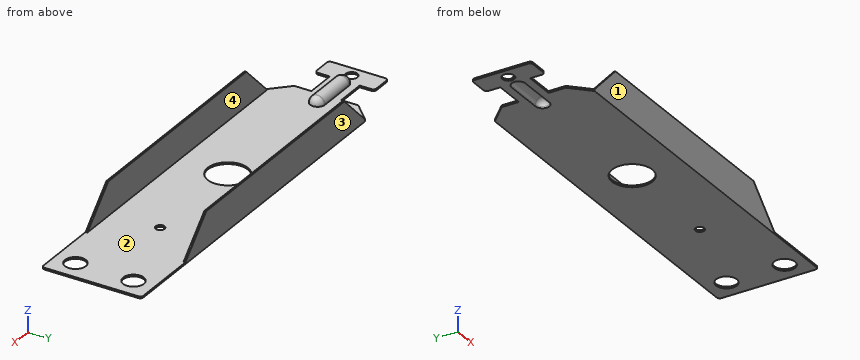
from build123d import *

# Parameters (mm, degrees)
F0_R     = 4.445
F0_R_2   = 8.5725
F0_R_3   = 1.905
F0_W     = 17.4625
F0_H     = 12.7
F0_W_2   = 12.7
F1_DEPTH = 0.762
F3_DEPTH = 0.762
F4_W     = 16.51
F4_H     = 2.921
F5_DEPTH = 25.4
F6_ANGLE = 180


# Not quite as in the source:
# - a pattern or mirror of a feature is missing from the dataset's text; its kind, count and spacing are read off the source's solid


with BuildPart() as f1:
    # F0 (on Top) → F1 (new body)
    with BuildSketch(Plane.XY):
        with BuildLine():
            Line((79.6925, 21.2725), (-73.3425, 21.2725))
            Line((-73.3425, 21.2725), (-80.9625, 13.6525))
            Line((-80.9625, 13.6525), (-80.9625, 6.35))
            Line((-80.9625, 6.35), (-63.5, 6.35))
            Line((-63.5, 6.35), (-63.5, -6.35))
            Line((-63.5, -6.35), (-80.9625, -6.35))
            Line((-80.9625, -6.35), (-80.9625, -13.6525))
            Line((-80.9625, -13.6525), (-73.3425, -21.2725))
            Line((-73.3425, -21.2725), (79.6925, -21.2725))
            ThreePointArc((79.6925, -21.2725), (80.5905256121, -20.9005256121), (80.9625, -20.0025))
            Line((80.9625, -20.0025), (80.9625, 20.0025))
            ThreePointArc((80.9625, 20.0025), (80.5905256121, 20.9005256121), (79.6925, 21.2725))
        make_face()
        with Locations((72.0725, -12.3825)):
            Circle(F0_R, mode=Mode.SUBTRACT)
        with Locations((-13.0175, 0)):
            Circle(F0_R_2, mode=Mode.SUBTRACT)
        with Locations((33.655, 0)):
            Circle(F0_R_3, mode=Mode.SUBTRACT)
        with Locations((72.0725, 12.3825)):
            Circle(F0_R, mode=Mode.SUBTRACT)
        with Locations((-72.23125, 0)):
            Rectangle(F0_W, F0_H)
        with Locations((-87.3125, 0)):
            Rectangle(F0_W_2, F0_H)
        with BuildLine():
            Line((-93.6625, -6.35), (-93.6625, 6.35))
            Line((-93.6625, 6.35), (-98.425, 6.35))
            Line((-98.425, 6.35), (-98.425, 2.54))
            ThreePointArc((-98.425, 2.54), (-96.6289487758, 1.7960512242), (-95.885, 0))
            ThreePointArc((-95.885, 0), (-96.6289487758, -1.7960512242), (-98.425, -2.54))
            Line((-98.425, -2.54), (-98.425, -6.35))
            Line((-98.425, -6.35), (-93.6625, -6.35))
        make_face()
        with BuildLine():
            Line((-98.425, 6.35), (-93.6625, 6.35))
            Line((-93.6625, 6.35), (-93.6625, 11.43))
            ThreePointArc((-93.6625, 11.43), (-94.0344743879, 12.3280256121), (-94.9325, 12.7))
            Line((-94.9325, 12.7), (-101.9175, 12.7))
            ThreePointArc((-101.9175, 12.7), (-102.8155256121, 12.3280256121), (-103.1875, 11.43))
            Line((-103.1875, 11.43), (-103.1875, -11.43))
            ThreePointArc((-103.1875, -11.43), (-102.8155256121, -12.3280256121), (-101.9175, -12.7))
            Line((-101.9175, -12.7), (-94.9325, -12.7))
            ThreePointArc((-94.9325, -12.7), (-94.0344743879, -12.3280256121), (-93.6625, -11.43))
            Line((-93.6625, -11.43), (-93.6625, -6.35))
            Line((-93.6625, -6.35), (-98.425, -6.35))
            Line((-98.425, -6.35), (-98.425, -2.54))
            ThreePointArc((-98.425, -2.54), (-100.965, 0), (-98.425, 2.54))
            Line((-98.425, 2.54), (-98.425, 6.35))
        make_face()
    extrude(amount=F1_DEPTH)

    # F2 (on face) → F3 (join)
    with BuildSketch(Plane.XZ.offset(21.2725)):
        Polygon((-58.9740902063, 15.1304097937), (-73.3425, 0.762), (50.6443195874, 0.762), (36.2759097937, 15.1304097937), align=None)
    f3 = extrude(amount=-F3_DEPTH)

    # F3_copies: F3 across plane
    add(f3.mirror(Plane.ZX))

    # F4 (on face) → F5 (cut)
    with BuildSketch(Plane.XY.offset(0.762)):
        with BuildLine():
            Line((-91.44, 0), (-91.44, 2.921))
            ThreePointArc((-91.44, 2.921), (-93.5054589078, 2.0654589078), (-94.361, 0))
            Line((-94.361, 0), (-91.44, 0))
        make_face()
        with BuildLine():
            Line((-91.44, -2.921), (-91.44, 0))
            Line((-91.44, 0), (-94.361, 0))
            ThreePointArc((-94.361, 0), (-93.5054589078, -2.0654589078), (-91.44, -2.921))
        make_face()
        with Locations((-83.185, 1.4605)):
            Rectangle(F4_W, F4_H)
        with BuildLine():
            Line((-72.009, 0), (-74.93, 0))
            Line((-74.93, 0), (-74.93, -2.921))
            ThreePointArc((-74.93, -2.921), (-72.8645410922, -2.0654589078), (-72.009, 0))
        make_face()
        with BuildLine():
            ThreePointArc((-72.009, 0), (-72.8645410922, 2.0654589078), (-74.93, 2.921))
            Line((-74.93, 2.921), (-74.93, 0))
            Line((-74.93, 0), (-72.009, 0))
        make_face()
        with Locations((-83.185, -1.4605)):
            Rectangle(F4_W, F4_H)
    extrude(amount=-F5_DEPTH, mode=Mode.SUBTRACT)

    # F4 (on face) → F6 (revolve)
    with BuildSketch(Plane.XY.offset(0.762)):
        with BuildLine():
            Line((-71.755, 0), (-72.009, 0))
            ThreePointArc((-72.009, 0), (-72.8645410922, -2.0654589078), (-74.93, -2.921))
            ThreePointArc((-74.93, -2.921), (-74.754023638, -2.9918379952), (-74.6762032813, -3.16484))
            ThreePointArc((-74.6762032813, -3.16484), (-72.5969301787, -2.1534646988), (-71.755, 0))
        make_face()
        with BuildLine():
            ThreePointArc((-74.6762032813, -3.16484), (-74.754023638, -2.9918379952), (-74.93, -2.921))
            Line((-74.93, -2.921), (-74.93, -3.175))
            ThreePointArc((-74.93, -3.175), (-74.803, -3.1724589832), (-74.6762032813, -3.16484))
        make_face()
        with BuildLine():
            Line((-74.93, -3.175), (-74.93, -2.921))
            ThreePointArc((-74.93, -2.921), (-75.1096051224, -2.9953948776), (-75.184, -3.175))
            Line((-75.184, -3.175), (-74.93, -3.175))
        make_face()
        with BuildLine():
            Line((-74.93, -2.921), (-91.44, -2.921))
            ThreePointArc((-91.44, -2.921), (-91.2603948776, -2.9953948776), (-91.186, -3.175))
            Line((-91.186, -3.175), (-75.184, -3.175))
            ThreePointArc((-75.184, -3.175), (-75.1096051224, -2.9953948776), (-74.93, -2.921))
        make_face()
        with BuildLine():
            ThreePointArc((-91.186, -3.175), (-91.2603948776, -2.9953948776), (-91.44, -2.921))
            Line((-91.44, -2.921), (-91.44, -3.175))
            Line((-91.44, -3.175), (-91.186, -3.175))
        make_face()
        with BuildLine():
            Line((-91.44, -3.175), (-91.44, -2.921))
            ThreePointArc((-91.44, -2.921), (-91.615976362, -2.9918379952), (-91.6937967187, -3.16484))
            ThreePointArc((-91.6937967187, -3.16484), (-91.567, -3.1724589832), (-91.44, -3.175))
        make_face()
        with BuildLine():
            ThreePointArc((-91.44, -2.921), (-93.5054589078, -2.0654589078), (-94.361, 0))
            Line((-94.361, 0), (-94.615, 0))
            ThreePointArc((-94.615, 0), (-93.7730698213, -2.1534646988), (-91.6937967187, -3.16484))
            ThreePointArc((-91.6937967187, -3.16484), (-91.615976362, -2.9918379952), (-91.44, -2.921))
        make_face()
    revolve(axis=Axis((-83.185, 0, 0.762), (-1, 0, 0)), revolution_arc=F6_ANGLE)


solid = f1.part
Model file for the job. Use its own axes, mm. Face numbers are marked on the shaded views. Give positions to 0.01 mm unless a question says otherwise; leave off trailing zeros. Loops run counter-clockwise (first coordinate to the right, second up) from the corner with the lowest first, then second, coordinate; pieces in that order, holes last. Notation, with made-up numbers: (-3, 72.25) -> (2, 72.25) arc R13 ccw to (2, 87.25) -> close; hole circle Ø8 at (-24.5, -26.75). An arc over 180 degrees is marked (long way). Use a Markdown table: item, result. Add a question column.
(1) Slice it at C-C on x = -20. List the corners of the cut face in (y, z).
(2) Slice it at B-B on x = -44.5. List the corners of the cut face in (y, z).
(3) Slice it at D-D on x = 69.5. List the corners of the cut face in (y, z).
(4) Wall check: line 1 along Y through (x, z) = (-56.5, 13); line 2 along Z through (x, y) = (-27, 19). Give the ranges that are in metal, low to high.
(5) Slice it at A-A on z = 13.25. List the corners of the cut face in (x, y), and give its area (3 significant figures).
(6) Drop flat-ended pins along their axis: pin 1 Ø19.5 at (x, y) = (-13.02, 0) entering from +Z; pin 2 Ø8 at (x, y) = (72.07, 12.38) entering from +Z; pin 3 Ø4 at (x, y) = (-78, 0.5) entering from -Z; pin 4 Ø0.6 at (x, z) = (-97, 0.5) entering from +Y. Give the stop position or say it passes through.
(7) Mould opens along Y. For the marked faces 1, 2, 3 and 4 say: +Y half, -Y half, draft (parallel to the pull), parting line (faces both ways), or undercut.
Filled sheet:
| question | item | result |
|---|---|---|
| 1 | outline | (-21.27, 0) -> (-4.97, 0) -> (-4.97, 0.76) -> (-20.51, 0.76) -> (-20.51, 15.13) -> (-21.27, 15.13) -> close; (4.97, 0) -> (21.27, 0) -> (21.27, 15.13) -> (20.51, 15.13) -> (20.51, 0.76) -> (4.97, 0.76) -> close |
| 2 | outline | (-21.27, 0) -> (21.27, 0) -> (21.27, 15.13) -> (20.51, 15.13) -> (20.51, 0.76) -> (-20.51, 0.76) -> (-20.51, 15.13) -> (-21.27, 15.13) -> close |
| 3 | outline | (-21.27, 0) -> (-16.01, 0) -> (-16.01, 0.76) -> (-21.27, 0.76) -> close; (-8.76, 0) -> (8.76, 0) -> (8.76, 0.76) -> (-8.76, 0.76) -> close; (16.01, 0) -> (21.27, 0) -> (21.27, 0.76) -> (16.01, 0.76) -> close |
| 4 | line 1 | -21.27 to -20.51, 20.51 to 21.27 |
| 4 | line 2 | 0 to 0.76 |
| 5 | outline | (-60.85, -21.27) -> (38.16, -21.27) -> (38.16, -20.51) -> (-60.85, -20.51) -> close; (-60.85, 20.51) -> (38.16, 20.51) -> (38.16, 21.27) -> (-60.85, 21.27) -> close |
| 5 | area | 151 mm2 |
| 6 | pin 1 | z = 0.76 |
| 6 | pin 2 | through |
| 6 | pin 3 | z = 2.27 |
| 6 | pin 4 | y = 12.7 |
| 7 | face 1 | -Y half |
| 7 | face 2 | undercut |
| 7 | face 3 | +Y half |
| 7 | face 4 | undercut |
